```python
from build123d import *

# Parameters (mm, degrees)
SKETCH_1_W          = 28.7
SKETCH_1_H          = 27.8
EXTRUDE_1_DEPTH     = 1.6
SKETCH_2_W          = 26.5
SKETCH_2_H          = 18.6
EXTRUDE_2_DEPTH     = 1.6
CUT_EXTRUDE_1_DEPTH = 21.042267836
CHAMFER_1_SIZE      = 0.5
SKETCH_4_W          = 10
SKETCH_4_H          = 2.5
EXTRUDE_3_DEPTH     = 2.5
SKETCH_5_W          = 8
SKETCH_5_H          = 1
EXTRUDE_4_DEPTH     = 5


with BuildPart() as part:
    # 草图1 → 凸台-拉伸1 (new body)
    with BuildSketch(Plane(origin=(0, 0, 0), x_dir=(1, 0, 0), z_dir=(0, 1, 0))):
        Rectangle(SKETCH_1_W, SKETCH_1_H)
    extrude(amount=EXTRUDE_1_DEPTH)

    # 草图2 → 凸台-拉伸2 (add)
    with BuildSketch(Plane(origin=(0, 1.6, 0), x_dir=(1, 0, 0), z_dir=(0, 1, 0))):
        Rectangle(SKETCH_2_W, SKETCH_2_H)
    extrude(amount=EXTRUDE_2_DEPTH)

    # 草图3 → 切除-拉伸1 (cut, through all)
    with BuildSketch(Plane(origin=(0, 1.6, 0), x_dir=(1, 0, 0), z_dir=(0, 1, 0))):
        with BuildLine():
            Line((-12, 12.9), (-10.6, 12.9))
            ThreePointArc((-10.6, 12.9), (-9.55, 11.85), (-10.6, 10.8))
            Line((-10.6, 10.8), (-12, 10.8))
            ThreePointArc((-12, 10.8), (-13.05, 11.85), (-12, 12.9))
        make_face()
        with BuildLine():
            Line((12, 12.9), (10.6, 12.9))
            ThreePointArc((10.6, 12.9), (9.55, 11.85), (10.6, 10.8))
            Line((10.6, 10.8), (12, 10.8))
            ThreePointArc((12, 10.8), (13.05, 11.85), (12, 12.9))
        make_face()
        with BuildLine():
            Line((12, -12.9), (10.6, -12.9))
            ThreePointArc((10.6, -12.9), (9.55, -11.85), (10.6, -10.8))
            Line((10.6, -10.8), (12, -10.8))
            ThreePointArc((12, -10.8), (13.05, -11.85), (12, -12.9))
        make_face()
        with BuildLine():
            Line((-12, -12.9), (-10.6, -12.9))
            ThreePointArc((-10.6, -12.9), (-9.55, -11.85), (-10.6, -10.8))
            Line((-10.6, -10.8), (-12, -10.8))
            ThreePointArc((-12, -10.8), (-13.05, -11.85), (-12, -12.9))
        make_face()
    extrude(amount=-CUT_EXTRUDE_1_DEPTH, mode=Mode.SUBTRACT)

    # 倒角1
    chamfer_1_edges = [part.edges().sort_by_distance(p)[0] for p in [
        (14.35, 0.8, 13.9),
        (-14.35, 0.8, 13.9),
        (-14.35, 0.8, -13.9),
        (14.35, 0.8, -13.9),
    ]]
    chamfer(chamfer_1_edges, length=CHAMFER_1_SIZE)

    # 草图4 → 凸台-拉伸3 (add)
    with BuildSketch(Plane.XZ):
        with Locations((0, 11.65)):
            Rectangle(SKETCH_4_W, SKETCH_4_H)
    extrude(amount=EXTRUDE_3_DEPTH)

    # 草图5 → 凸台-拉伸4 (add)
    with BuildSketch(Plane.XZ.offset(2.5)):
        with Locations((-0.103219582, 11.669441564)):
            Rectangle(SKETCH_5_W, SKETCH_5_H)
    extrude(amount=EXTRUDE_4_DEPTH)


solid = part.part
```
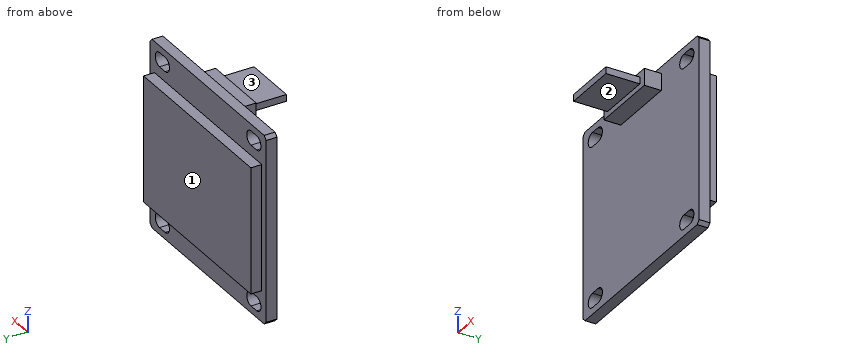
Design review of the part built by this model. Coordinates are the model's own, in mm. Face numbers are marked on the shaded views. A direction names the side the tool comes from. Give positions to 0.01 mm unless a question says otherwise; leave off trailing zeros. Order: outer loops, then holes, each group sorted by start corner. A loop starts at its lowest first (then second) coordinate and runs counter-clockwise, first axis right, second up. Notation, with made-up numbers: (-17, 81.25) -> (-10, 81.25) arc R28 cw to (-10, 100.25) -> close; hole circle Ø4 at (-25, 71.5). An arc over 180 degrees is marked (long way). Write item = value, one per line. Start each with the question number.
(1) We need section B-B on y = 1.25. Write out the cut boundary in (x, z), plus the area to 3 significant figures.
(2) For the marked faces 1, 2 and 3, list the 3-axis set-ups (+Z, -Z, +X, -X, +Y, -Y) from which the entire face can be reached by the end or side of a thin tool; tool diameter is ignored.
(3) We need section D-D on z = 8.5. Write out the cut boundary in (x, y).
(4) For pin 1 (0.5 mm diameter, centred on y = 2, z = -4.5, fed in from +X); pin 2 (1.5 mm diameter, centred on x = -0.5, y = -5.5, fed in from -Z); pin 3 (1 mm diameter, centred on x = -7.5, z = 8, fed in from -Y); pin 4 (5 mm diameter, centred on y = -1, z = 0, fed in from -X), all flat-tipped, find the tip position at first contact; note any pin that passes through.
(5) To check wall thickness, follow line 1 along Y through (x, z) = (-12.5, 8.75); line 2 along Y through (x, z) = (-3.75, -9.5); line 3 along Z through (x, y) = (-0.25, -3.5). State the ranges of each line that lie inside material, in increasing order.
(6) We need section C-C on x = -2.5. Write out the cut boundary in (y, z).
(7) We need section A-A on x = -11.25. Write out the cut boundary in (y, z), plus the area to 3 significant figures.
Numbers:
q1.outline = (-14.35, -13.4) -> (-13.85, -13.9) -> (13.85, -13.9) -> (14.35, -13.4) -> (14.35, 13.4) -> (13.85, 13.9) -> (-13.85, 13.9) -> (-14.35, 13.4) -> close; hole (-12, -12.9) -> (-10.6, -12.9) arc R1.05 ccw to (-10.6, -10.8) -> (-12, -10.8) arc R1.05 ccw to start; hole (-12, 10.8) -> (-10.6, 10.8) arc R1.05 ccw to (-10.6, 12.9) -> (-12, 12.9) arc R1.05 ccw to start; hole (10.6, -12.9) -> (12, -12.9) arc R1.05 ccw to (12, -10.8) -> (10.6, -10.8) arc R1.05 ccw to start; hole (10.6, 10.8) -> (12, 10.8) arc R1.05 ccw to (12, 12.9) -> (10.6, 12.9) arc R1.05 ccw to start
q1.area = 772 mm^2
q2.face_1 = +Z, -Z, +X, -X, +Y
q2.face_2 = -Z, +X, -X, -Y
q2.face_3 = +Z, +X, -X, -Y
q3.outline = (-14.35, 0) -> (14.35, 0) -> (14.35, 1.6) -> (13.25, 1.6) -> (13.25, 3.2) -> (-13.25, 3.2) -> (-13.25, 1.6) -> (-14.35, 1.6) -> close
q4.pin_1 = 13.25
q4.pin_2 = 11.17
q4.pin_3 = 0
q4.pin_4 = -14.35
q5.line_1 = 0 to 3.2
q5.line_2 = 0 to 1.6
q5.line_3 = 11.17 to 12.17
q6.outline = (-7.5, 11.17) -> (-2.5, 11.17) -> (-2.5, 10.4) -> (0, 10.4) -> (0, -13.9) -> (1.6, -13.9) -> (1.6, -9.3) -> (3.2, -9.3) -> (3.2, 9.3) -> (1.6, 9.3) -> (1.6, 13.9) -> (0, 13.9) -> (0, 12.9) -> (-2.5, 12.9) -> (-2.5, 12.17) -> (-7.5, 12.17) -> close
q7.outline = (0, -13.9) -> (1.6, -13.9) -> (1.6, -12.9) -> (0, -12.9) -> close; (0, -10.8) -> (1.6, -10.8) -> (1.6, -9.3) -> (3.2, -9.3) -> (3.2, 9.3) -> (1.6, 9.3) -> (1.6, 10.8) -> (0, 10.8) -> close; (0, 12.9) -> (1.6, 12.9) -> (1.6, 13.9) -> (0, 13.9) -> close
q7.area = 67.5 mm^2
